```python
from build123d import *

# Parameters (mm, degrees)
SKETCH2_W          = 101.6
SKETCH2_H          = 101.6
CUT_EXTRUDE1_DEPTH = 17.78


with BuildPart() as part:
    # Sketch1 → Revolve1 (revolve)
    with BuildSketch(Plane.XY):
        with BuildLine():
            Line((0, 0), (228.6, 0))
            ThreePointArc((228.6, 0), (161.644610179, 161.644610179), (0, 228.6))
            Line((0, 228.6), (0, 0))
        make_face()
    revolve(axis=Axis((0, 0, 0), (0, 1, 0)))

    # Sketch2 → Cut-Extrude1 (cut)
    with BuildSketch(Plane(origin=(0, 228.6, 0), x_dir=(1, 0, 0), z_dir=(0, 1, 0))):
        Rectangle(SKETCH2_W, SKETCH2_H)
    extrude(amount=-CUT_EXTRUDE1_DEPTH, mode=Mode.SUBTRACT)


solid = part.part
```
Can you work these out from the model? Positions are in its coordinate system, mm. Round coordinates to 2 decimals unless told otherwise and drop trailing zeros. Loops run counter-clockwise (first coordinate to the right, second up) from the corner with the lowest first, then second, coordinate; pieces in that order, holes last.
Item 1: If we mould it in two halves opening along X, with no side actions, what happens to faces 1 (the flat face through (3, 0, -3)), 2 (the flat face through (-50.8, 216, 1))? For each: +X half, -X half, draft (parallel to the pull), parting line (faces both ways), or undercut.
Item 2: Suppose I cut it at D-D, the plane x = 152. Write out the boundary of the cut face in (y, z).
Item 3: Please list where these lines run through material, in increasing order: L1, parallel to Y at x = 19, z = 8.5; L2, parallel to Z at x = -122.5, y = 124.5; L3, parallel to Z at x = 51, y = 48.5.
Item 4: Suppose I cut it at B-B, the plane y = 161. Write out the boundary of the cut face in (x, z), then the cut area to 3 significant figures.
Item 5: Suppose I cut it at A-A, the plane x = 9.5. Write out the boundary of the cut face in (y, z).
Item 6: Suppose I cut it at C-C, the plane z = 127. Write out the boundary of the cut face in (x, y), then the cut area to 3 significant figures.
Item 7: Will these pins go through, and if not, where does the flat tip stop? pin 1 Ø5 at (x, z) = (11.5, 172.5) entering from +Y; pin 2 Ø6 at (x, y) = (6, 214) entering from -Z; pin 3 Ø12 at (x, z) = (-0.5, -85) entering from +Y.
Reported:
1. face 1: draft
1. face 2: undercut
2. outline: (0, -170.75) arc R170.75 ccw to (0, 170.75) - close
3. L1: y = 0 to 210.82
3. L2: z = -147.48 to 147.48
3. L3: z = -217.5 to 217.5
4. outline: circle Ø324.57 at (0, 0)
4. area: 82,700 mm2
5. outline: (0, -228.4) arc R228.4 ccw to (222.68, -50.8) - (210.82, -50.8) - (210.82, 50.8) - (222.68, 50.8) arc R228.4 ccw to (0, 228.4) - close
6. outline: (-190.08, 0) - (190.08, 0) arc R190.08 ccw to start
6. area: 56,800 mm2
7. pin 1: stops at y = 152.41
7. pin 2: stops at z = -87.76
7. pin 3: stops at y = 214.52
